Source: CAD feature listing. Evaluate the final solid. Frame: model axes, mm. Face numbers are marked on the shaded views. Give positions to 0.01 mm unless a question says otherwise; leave off trailing zeros. Order: outer loops, then holes, each group sorted by start corner. A loop starts at its lowest first (then second) coordinate and runs counter-clockwise, first axis right, second up. Notation, with made-up numbers: M 6,29.25 L 24,29.25 A20 cw 24,46.25 Z; hole C -24,2 d10. An arc over 180 degrees is marked long. Return JSON: item names as keys, results as strings.
Autodesk Inventor part; units mm, degrees
ref_plane "YZ Plane" through (0, 0, 0) normal (1, 0, 0) x (0, 1, 0)
ref_plane "XZ Plane" through (0, 0, 0) normal (0, 1, 0) x (-1, 0, 0)
ref_plane "XY Plane" through (0, 0, 0) normal (0, 0, 1) x (1, 0, 0)
sketch "Sketch1" plane through (0, 0, 0) normal (1, 0, 0) x (0, 1, 0)
  line L0 (0, 0.9489) -> (25.4, 0.9489)
  line L1 (25.4, 0.9489) -> (25.4, 77.1489)
  line L2 (25.4, 77.1489) -> (0, 77.1489)
  line L3 (0, 77.1489) -> (0, 0.9489)
  point P0 (0, 0)
  dimension "d0" = 25.4
  dimension "d1" = 76.2
extrude "Extrusion1" add sketch "Sketch1" along normal blind 12.7
sketch "Sketch2" plane through (0, 0, 0) normal (-1, 0, 0) x (0, 0, 1)
  line L0 (77.1489, 25.4) -> (77.1489, 0)
  line L1 (0.9489, 25.4) -> (77.1489, 25.4)
  point P0 (0, 0)
  point P1 (64.4489, 12.7)
  dimension "d4" = 12.7
  dimension "d5" = 12.7
hole "Hole1" at (0, 12.7, 64.4489) direction (1, 0, 0) diameter 12.7 end through all
fillet "Fillet1" radius 12.7 2 edges at (6.35, 25.4, 77.1489) (6.35, 0, 77.1489)
sketch "Sketch3" plane through (0, 0, 0) normal (-1, 0, 0) x (0, 0, 1)
  line L0 (0.9489, 25.4) -> (64.4489, 25.4)
  line L1 (0.9489, 0) -> (0.9489, 25.4)
  line L2 (64.4489, 0) -> (0.9489, 0)
  line L3 (0.9489, 20.6375) -> (43.8114, 20.6375)
  line L4 (43.8114, 4.7625) -> (0.9489, 4.7625)
  line L5 (0.9489, 4.7625) -> (0.9489, 20.6375)
  arc A0 (43.8114, 7.9375) -> (43.8114, 17.4625) centre (43.8114, 12.7) ccw
  line L6 (43.8114, 20.6375) -> (43.8114, 17.4625)
  line L7 (43.8114, 7.9375) -> (43.8114, 4.7625)
  point P0 (0, 0)
  dimension "d15" = 4.7625
  dimension "d16" = 4.7625
  dimension "d18" = 3.175
  dimension "d19" = 3.175
  dimension "d20" = 4.7625
  dimension "d21" = 42.8625
extrude "Extrusion2" cut sketch "Sketch3" against normal through all
sketch "Sketch4" plane through (0, 0, 0.9489) normal (0, -1, 0) x (1, 0, 0)
  line L0 (0, 0) -> (12.7, 0)
  circle A0 centre (6.35, 12.7) radius 9.525
  line L1 (12.7, 63.5) -> (12.7, 0)
  point P0 (0, -0.9489)
  dimension "d24" = 12.7
  dimension "d25" = 19.05
  dimension "d49" = 6.35
extrude "Extrusion3" add sketch "Sketch4" along normal up to surface (4.7625 mm away) from surface at -4.7625
sketch "Sketch5" plane through (0, 25.4, 0.9489) normal (0, 1, 0) x (1, 0, 0)
  circle A0 centre (5.5563, -12.7) radius 9.525
  point P0 (12.7, 0)
  point P1 (0, 0.9489)
  dimension "d28" = 19.05
  dimension "d29" = 12.7
extrude "Extrusion4" add sketch "Sketch5" along normal up to surface (4.7625 mm away) from surface at -4.7625
sketch "Sketch6" plane through (0, 25.4, 0.9489) normal (0, 1, 0) x (1, 0, 0)
  arc A0 (12.7, -19.0002) -> (12.7, -6.3998) centre (5.5563, -12.7) ccw
  circle A1 centre (5.5563, -12.7) radius 7.1438
  point P0 (0, 0.9489)
  dimension "d32" = 14.2875
extrude "Extrusion5" add sketch "Sketch6" along normal blind 0.7937 and the other way blind 5.5563
sketch "Sketch7" plane through (0, 0, 0.9489) normal (0, -1, 0) x (1, 0, 0)
  arc A0 (12.7, 5.6005) -> (12.7, 19.7995) centre (6.35, 12.7) ccw
  circle A1 centre (6.35, 12.7) radius 7.1437
  point P0 (0, -0.9489)
  dimension "d37" = 14.2875
extrude "Extrusion6" add sketch "Sketch7" along normal blind 0.7937 and the other way blind 5.5563
sketch "Sketch8" plane through (6.35, -0.7938, 13.6489) normal (0, -1, 0) x (1, 0, 0)
  circle A0 centre (0, 0) radius 7.1437
  point P0 (-6.35, -13.6489)
hole "Hole2" at (6.35, -0.7938, 13.6489) direction (0, 1, 0) diameter 6.35 end through all
properties part number "pulley hook" material "Acetal Resin, Black"
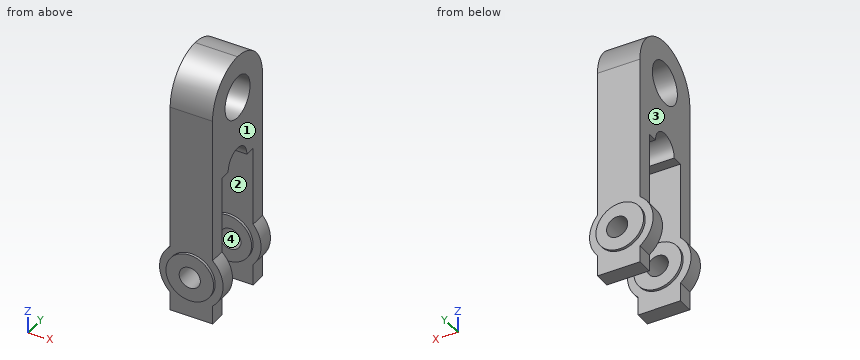
1. Draft query along X for the marked faces 1, 2, 3 and 4. Return one class per face: pulls with the +X half, pulls with the -X half, needs draft (parallel to the pull), parting line crosses it, or undercut.
Evaluation:
{"face 1": "pulls with the +X half", "face 2": "needs draft", "face 3": "pulls with the -X half", "face 4": "undercut"}
2. Section query C-C (y = 22). Return loops of the section in (x, z) (3 decimals), then the cut area to 3 significant figures.
Evaluation:
{"outline": "M 0,0.949 L 12.7,0.949 L 12.7,7.349 A9.525 ccw 12.7,19.949 L 12.7,73.098 L 0,73.098 L 0,21.385 A9.525 ccw 0,5.912 Z; hole C 6.35,13.649 d6.35", "area": "948 mm^2"}
3. Section query B-B (y = 10.75). Return loops of the section in (x, z).
Evaluation:
{"outline": "M 0,48.16 L 12.7,48.16 L 12.7,58.41 L 0,58.41 Z; M 0,70.49 L 12.7,70.49 L 12.7,77 L 0,77 Z"}
4. Ray query, probe 1 along Y at (x, z) = (4.75, 35.5); probe 2 along Y at (x, z) = (10.75, 19); probe 3 along X at (y, z) = (6.75, 52). Return the intervals inside material, ascending.
Evaluation:
{"probe 1": "y = 0 to 4.76, 20.64 to 25.4", "probe 2": "y = -0.79 to 5.56, 20.64 to 25.4", "probe 3": "x = 0 to 12.7"}
5. Section query A-A (z = 28). Return loops of the section in (x, y).
Evaluation:
{"outline": "M 0,0 L 12.7,0 L 12.7,4.76 L 0,4.76 Z; M 0,20.64 L 12.7,20.64 L 12.7,25.4 L 0,25.4 Z"}
6. First-contact query: pin 1 (12 mm diameter, centred on y = 9.5, z = 25, fed in from -X); pin 2 (10 mm diameter, centred on x = 11, y = 3, fed in from +Z); pin 3 (5.5 mm diameter, centred on x = 7.5, z = 40, fed in from +Y). Flat tips, straight axial feed; report the tip coordinate or a pass-through.
Evaluation:
{"pin 1": "stops at x = 0", "pin 2": "stops at z = 76.25", "pin 3": "stops at y = 25.4"}
7. Section query D-D (x = 6.35). State how many separate pieces and enclosed holes the cut face has, then the cut area to 3 significant figures.
Evaluation:
{"separate pieces": "3", "enclosed holes": "1", "area": "988 mm^2"}
